Geometry: final body of the model. Coordinates: model frame, mm. Face numbers are marked on the shaded views. A direction names the side the tool comes from. Give positions to 0.01 mm unless a question says otherwise; leave off trailing zeros. Write each loop counter-clockwise with the first axis right and the second up, starting at its lowest first coordinate (ties: lowest second). Pieces come first, ordered by that corner, then holes. Notation, with made-up numbers: M -24,-12.75 L 10,-12.75 A24 cw 10,26.25 Z; hole C 46,2 d2. An arc over 180 degrees is marked long. Answer as a JSON object with one key per item and string values.
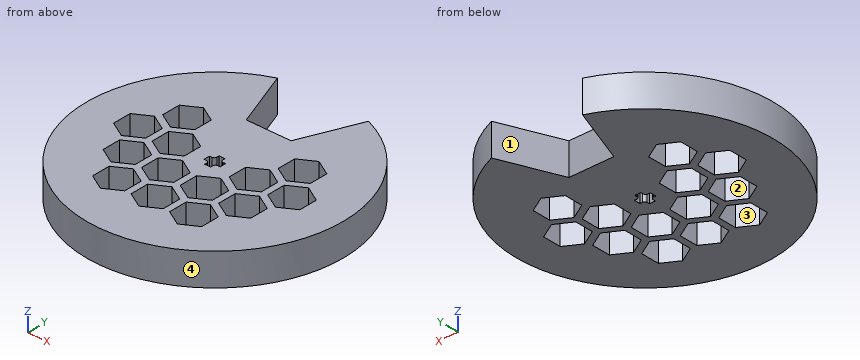
from build123d import *

# Parameters (mm, degrees)
SKETCH1_R                = 40
BOSS_EXTRUDE1_DEPTH      = 10
CUT_EXTRUDE8_DEPTH       = 99
CUT_EXTRUDE9_DEPTH       = 58.445626465
CUT_EXTRUDE9_DEPTH_BACK  = 58.445626465
CUT_EXTRUDE10_DEPTH      = 23
CUT_EXTRUDE10_DEPTH_BACK = 58.445626465


with BuildPart() as part:
    # Sketch1 → Boss-Extrude1 (new body)
    with BuildSketch(Plane.XY):
        Circle(SKETCH1_R)
    extrude(amount=BOSS_EXTRUDE1_DEPTH)

    # Sketch1<10> → Cut-Extrude8 (cut)
    with BuildSketch(Plane.XY):
        Polygon((17, 2.886751346), (12, 5.773502692), (7, 2.886751346), (7, -2.886751346), (12, -5.773502692), (17, -2.886751346), align=None)
        Polygon((29, 2.886751346), (24, 5.773502692), (19, 2.886751346), (19, -2.886751346), (24, -5.773502692), (29, -2.886751346), align=None)
        Polygon((-7, 2.886751346), (-12, 5.773502692), (-17, 2.886751346), (-17, -2.886751346), (-12, -5.773502692), (-7, -2.886751346), align=None)
        Polygon((-19, 2.886751346), (-24, 5.773502692), (-29, 2.886751346), (-29, -2.886751346), (-24, -5.773502692), (-19, -2.886751346), align=None)
        Polygon((-13, 13.279056191), (-18, 16.165807537), (-23, 13.279056191), (-23, 7.505553499), (-18, 4.618802154), (-13, 7.505553499), align=None)
        Polygon((23, 7.505553499), (23, 13.279056191), (18, 16.165807537), (13, 13.279056191), (13, 7.505553499), (18, 4.618802154), align=None)
        Polygon((-13, -13.279056191), (-13, -7.505553499), (-18, -4.618802154), (-23, -7.505553499), (-23, -13.279056191), (-18, -16.165807537), align=None)
        Polygon((-11, -13.279056191), (-6, -16.165807537), (-1, -13.279056191), (-1, -7.505553499), (-6, -4.618802154), (-11, -7.505553499), align=None)
        Polygon((6, -16.165807537), (11, -13.279056191), (11, -7.505553499), (6, -4.618802154), (1, -7.505553499), (1, -13.279056191), align=None)
        Polygon((13, -7.505553499), (13, -13.279056191), (18, -16.165807537), (23, -13.279056191), (23, -7.505553499), (18, -4.618802154), align=None)
        Polygon((-17, -23.671361037), (-12, -26.558112383), (-7, -23.671361037), (-7, -17.897858345), (-12, -15.011106999), (-17, -17.897858345), align=None)
        Polygon((0, -26.558112383), (5, -23.671361037), (5, -17.897858345), (0, -15.011106999), (-5, -17.897858345), (-5, -23.671361037), align=None)
        Polygon((7, -17.897858345), (7, -23.671361037), (12, -26.558112383), (17, -23.671361037), (17, -17.897858345), (12, -15.011106999), align=None)
    extrude(amount=CUT_EXTRUDE8_DEPTH, mode=Mode.SUBTRACT)

    # Sketch1<11> → Cut-Extrude9 (cut, two sides: drawn at the far end of the back side and taken through both)
    with BuildSketch(Plane.XY.offset(-CUT_EXTRUDE9_DEPTH_BACK)):
        with BuildLine():
            Line((-6.994087027, 18.73720221), (0, 18.73720221))
            Line((0, 18.73720221), (7.005912973, 18.73720221))
            Line((7.005912973, 18.73720221), (14.620716001, 37.232172427))
            ThreePointArc((14.620716001, 37.232172427), (0.338668589, 39.998566269), (-13.988174054, 37.47440442))
            Line((-13.988174054, 37.47440442), (-6.994087027, 18.73720221))
        make_face()
    extrude(amount=CUT_EXTRUDE9_DEPTH + CUT_EXTRUDE9_DEPTH_BACK, mode=Mode.SUBTRACT)

    # Sketch1<13> → Cut-Extrude10 (cut, two sides: drawn at the far end of the back side and taken through both)
    with BuildSketch(Plane.XY.offset(-CUT_EXTRUDE10_DEPTH_BACK)):
        with BuildLine():
            Line((0.853688676, -2.457553929), (-1.020561324, -2.457553929))
            Line((-1.020561324, -2.457553929), (-1.020561324, -1.672692112))
            ThreePointArc((-1.020561324, -1.672692112), (-1.25214669, -1.114915123), (-1.810695088, -0.885196516))
            Line((-1.810695088, -0.885196516), (-2.590311324, -0.887803929))
            Line((-2.590311324, -0.887803929), (-2.590311324, 0.991696071))
            Line((-2.590311324, 0.991696071), (-1.802811324, 0.991696071))
            ThreePointArc((-1.802811324, 0.991696071), (-1.245964734, 1.222349481), (-1.015311324, 1.779196071))
            Line((-1.015311324, 1.779196071), (-1.015311324, 2.561446071))
            Line((-1.015311324, 2.561446071), (0.858938676, 2.561446071))
            Line((0.858938676, 2.561446071), (0.858938676, 1.776584255))
            ThreePointArc((0.858938676, 1.776584255), (1.090524042, 1.218807266), (1.649072441, 0.989088659))
            Line((1.649072441, 0.989088659), (2.428688676, 0.991696071))
            Line((2.428688676, 0.991696071), (2.428688676, -0.887803929))
            Line((2.428688676, -0.887803929), (1.641188676, -0.887803929))
            ThreePointArc((1.641188676, -0.887803929), (1.084342086, -1.118457338), (0.853688676, -1.675303929))
            Line((0.853688676, -1.675303929), (0.853688676, -2.457553929))
        make_face()
    extrude(amount=CUT_EXTRUDE10_DEPTH + CUT_EXTRUDE10_DEPTH_BACK, mode=Mode.SUBTRACT)


solid = part.part
1) Pull-direction query (X, two-part tool) for the marked faces 3 and 4; classes: pulls with the +X half, pulls with the -X half, needs draft (parallel to the pull), parting line crosses it, or undercut.
Geometry check:
{"face 3": "undercut", "face 4": "parting line crosses it"}
2) Set-up query: the marked faces 1 and 2. Return all of +Z, -Z, +X, -X, +Y, -Y with unobstructed straight access to the full face (end or side cutting, diameter ignored); none if empty.
Geometry check:
{"face 1": "+Z, -Z, +Y", "face 2": "+Z, -Z"}
3) Cut plane D-D on z = 2.75. Give the number of separate pieces and of enclosed holes in the cut face, and give its area (3 significant figures).
Geometry check:
{"separate pieces": "1", "enclosed holes": "14", "area": "3,440 mm2"}
4) Cut plane B-B on x = 8.5. Return loops of the section in (y, z), and give its area (3 significant figures).
Geometry check:
{"outline": "M -39.09,0 L -24.54,0 L -24.54,10 L -39.09,10 Z; M -17.03,0 L -14.72,0 L -14.72,10 L -17.03,10 Z; M -6.06,0 L -3.75,0 L -3.75,10 L -6.06,10 Z; M 3.75,0 L 22.37,0 L 22.37,10 L 3.75,10 Z", "area": "378 mm2"}
5) Line query: line 1 (Y direction, x = -0.5, z = 9); line 2 (X direction, y = 2, z = 5.25); line 3 (X direction, y = -24, z = 4.5). Output: solid intervals per line, ascending. Write a range as from..to.
Geometry check:
{"line 1": "y = -40..-26.27, -15.3..-2.46, 2.56..18.74", "line 2": "x = -39.95..-29, -19..-17, -7..-1.02, 0.86..7, 17..19, 29..39.95", "line 3": "x = -32..-16.43, -7.57..-4.43, 4.43..7.57, 16.43..32"}
6) Contact query for flat-ended pins moving along their axis: P1, Ø3, axis at y = -22, z = 3.5, coming from the +X side; P2, Ø5, axis at x = -26, z = 8.5, coming from the +Y side; P3, Ø3, axis at y = -24.5, z = 7, coming from the +X side. Output: stop coordinate, or through.
Geometry check:
{"P1": "stops at x = 34.35", "P2": "stops at y = 32.37", "P3": "stops at x = 32.73"}
7) Cut plane A-A on y = 9.5. Return loops of the section in (x, z).
Geometry check:
{"outline": "M -38.86,0 L -23,0 L -23,10 L -38.86,10 Z; M -13,0 L 13,0 L 13,10 L -13,10 Z; M 23,0 L 38.86,0 L 38.86,10 L 23,10 Z"}
8) Cut plane C-C on y = 23. Return loops of the section in (x, z), and give its area (3 significant figures).
Geometry check:
{"outline": "M -32.73,0 L -8.59,0 L -8.59,10 L -32.73,10 Z; M 8.76,0 L 32.73,0 L 32.73,10 L 8.76,10 Z", "area": "481 mm2"}
